Build history of the part. All positions in model axes, mm. Face numbers are marked on the shaded views. Round coordinates to 2 decimals unless told otherwise and drop trailing zeros. Order: outer loops, then holes, each group sorted by start corner. A loop starts at its lowest first (then second) coordinate and runs counter-clockwise, first axis right, second up. Notation, with made-up numbers: (-37, 86.25) -> (19, 86.25) arc R9 ccw to (19, 103.25) -> close; hole circle Ø7 at (57, -20.75). An arc over 180 degrees is marked (long way). Answer as a JSON object with one key per item and string values.
from build123d import *

# Parameters (mm, degrees)
F0_R      = 2.555
F0_R_2    = 1.475
F1_DEPTH  = 2.41
F2_W      = 1.46
F2_H      = 2.11
F3_DEPTH  = 2.1
F5_DEPTH  = 25
F7_DEPTH  = 25
F9_DEPTH  = 25
F10_R     = 5.425
F10_R_2   = 4.549258
F11_DEPTH = 0.99
F12_R     = 0.33799


with BuildPart() as f1:
    # F0 (on Front) → F1 (new body)
    with BuildSketch(Plane.XZ):
        Circle(F0_R)
        Circle(F0_R_2, mode=Mode.SUBTRACT)
    extrude(amount=F1_DEPTH)

    # F2 (on face) → F3 (join)
    with BuildSketch(Plane.XZ.offset(2.41)):
        with Locations((0, 3.503494)):
            Rectangle(F2_W, F2_H)
        Polygon((-3.582772, -2.911446), (-1.755458, -1.856446), (-2.485458, -0.592049), (-4.312772, -1.647049), align=None)
        Polygon((4.312772, -1.647049), (2.485458, -0.592049), (1.755458, -1.856446), (3.582772, -2.911446), align=None)
    extrude(amount=-F3_DEPTH)

    # F4 (on face) → F5 (cut)
    with BuildSketch(Plane(origin=(-0.365, 0, -0.632199), x_dir=(0.866025, 0, -0.5), z_dir=(-0.5, 0, -0.866025))):
        Polygon((4.558494, 1.42), (2.448494, 0.31), (3.479598, 0.083374), (4.896949, 0.210857), (4.896949, 2.56652), (4.714418, 2.478824), (4.714418, 1.641871), align=None)
    extrude(amount=-F5_DEPTH, mode=Mode.SUBTRACT)

    # F6 (on face) → F7 (cut)
    with BuildSketch(Plane(origin=(-0.73, 0, 0), x_dir=(0, -1, 0), z_dir=(-1, 0, 0))):
        Polygon((0.091005, 3.516779), (0.31, 2.448494), (1.42, 4.558494), (2.41, 4.741723), (0.190774, 5.01886), align=None)
    extrude(amount=-F7_DEPTH, mode=Mode.SUBTRACT)

    # F8 (on face) → F9 (cut)
    with BuildSketch(Plane(origin=(0.365, 0, -0.632199), x_dir=(0.866025, 0, 0.5), z_dir=(0.5, 0, -0.866025))):
        Polygon((-4.558494, 1.42), (-5.496076, 1.436378), (-4.840972, -0.092841), (-2.670947, -0.092841), (-2.448494, 0.31), align=None)
    extrude(amount=-F9_DEPTH, mode=Mode.SUBTRACT)

    # F10 (on face) → F11 (join)
    with BuildSketch(Plane.XZ.offset(2.41)):
        Circle(F10_R)
        Circle(F10_R_2, mode=Mode.SUBTRACT)
    extrude(amount=-F11_DEPTH)

    # F12
    f12_edges = [f1.edges().sort_by_distance(p)[0] for p in [
        (-5.425, -2.41, 0),
    ]]
    fillet(f12_edges, radius=F12_R)


solid = f1.part
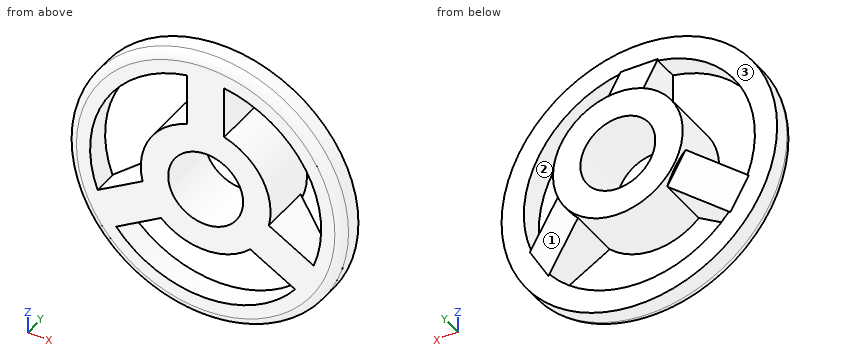
1) Probe L1, parallel to Z at x = 0, y = -1.7 (3 decimals); L2, parallel to Z at x = -3.25, y = -2.1; L3, parallel to Z at x = 1, y = -1.6. List the from-to ranges inside material, lowest first. Write a range as from..to.
Checked values:
{"L1": "z = -5.425..-4.549, -2.555..-1.475, 1.475..5.425", "L2": "z = -4.34..-3.18, -2.72..-1.03, 3.18..4.34", "L3": "z = -5.33..-4.44, -2.35..-1.08, 1.08..2.35, 4.44..5.33"}
2) Cut at A-A, the plane x = 0. Count the separate pieces of the cut face and the enclosed holes in it, plus the area to 3 significant figures.
Checked values:
{"separate pieces": "3", "enclosed holes": "0", "area": "9.92 mm²"}
3) Flat gauge pins, fed straight in: pin 1 Ø6 at (x, z) = (2.5, -3.5) entering from -Y; pin 2 Ø2 at (x, z) = (4, -0.5) entering from +Y; pin 3 Ø1 at (y, z) = (-1.5, 3.5) entering from +X. Where does each tip first touch, or does it go through?
Checked values:
{"pin 1": "stops at y = -2.41", "pin 2": "stops at y = -0.69", "pin 3": "stops at x = 4.52"}
4) Cut at B-B, the plane z = 0. Give the cut face in (x, y) (3 decimals).
Checked values:
{"outline": "(-5.425, -2.072) arc R0.338 ccw to (-5.087, -2.41) -> (-4.549, -2.41) -> (-4.549, -1.42) -> (-5.425, -1.42) -> close; (-2.555, -2.41) -> (-1.475, -2.41) -> (-1.475, 0) -> (-2.555, 0) -> close; (1.475, -2.41) -> (2.555, -2.41) -> (2.555, 0) -> (1.475, 0) -> close; (4.549, -2.41) -> (5.087, -2.41) arc R0.338 ccw to (5.425, -2.072) -> (5.425, -1.42) -> (4.549, -1.42) -> close"}
5) Pull direction X, two halves, no side cores. Call the marked faces 1, 2 and 3: pulls with the +X half, pulls with the -X half, needs draft (parallel to the pull), parting line crosses it, or undercut.
Checked values:
{"face 1": "pulls with the +X half", "face 2": "undercut", "face 3": "needs draft"}
